Design review of the part built by this model. Coordinates are the model's own, in mm. Face numbers are marked on the shaded views. A direction names the side the tool comes from. Give positions to 0.01 mm unless a question says otherwise; leave off trailing zeros. Loops run counter-clockwise (first coordinate to the right, second up) from the corner with the lowest first, then second, coordinate; pieces in that order, holes last. Notation, with made-up numbers: M 64.25,73.5 L 87.25,73.5 A34 ccw 87.25,108.5 Z; hole C 56.25,12.25 d4. An arc over 180 degrees is marked long. Answer as CSV lines item,"result".
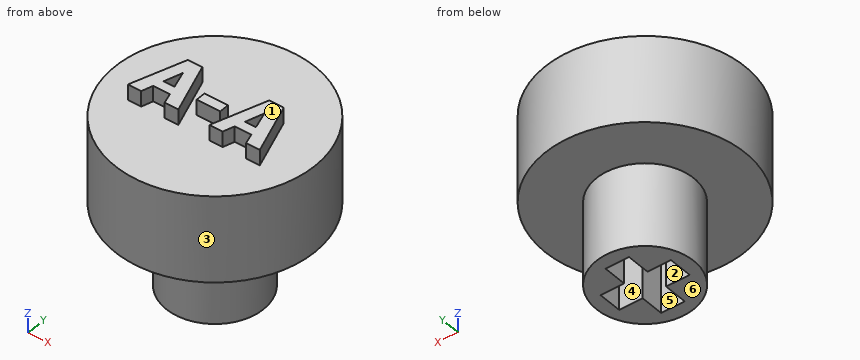
Autodesk Inventor part; units mm, degrees
ref_plane "YZ Plane" through (0, 0, 0) normal (1, 0, 0) x (0, 1, 0)
ref_plane "XZ Plane" through (0, 0, 0) normal (0, 1, 0) x (-1, 0, 0)
ref_plane "XY Plane" through (0, 0, 0) normal (0, 0, 1) x (1, 0, 0)
sketch "Sketch1" plane through (0, 0, 0) normal (0, 0, 1) x (1, 0, 0)
  circle A0 centre (0, 0) radius 6.22 construction
  circle A1 centre (0, 0) radius 2.8
  line L0 (-0.675, 0.675) -> (-0.675, 2.025)
  line L1 (-0.675, 2.025) -> (0.675, 2.025)
  line L2 (0.675, 2.025) -> (0.675, 0.675)
  line L3 (0.675, 0.675) -> (2.025, 0.675)
  line L4 (2.025, 0.675) -> (2.025, -0.675)
  line L5 (2.025, -0.675) -> (0.675, -0.675)
  line L6 (0.675, -0.675) -> (0.675, -2.025)
  line L7 (0.675, -2.025) -> (-0.675, -2.025)
  line L8 (-0.675, -2.025) -> (-0.675, -0.675)
  line L9 (-0.675, -0.675) -> (-2.025, -0.675)
  line L10 (-2.025, -0.675) -> (-2.025, 0.675)
  line L11 (-2.025, 0.675) -> (-0.675, 0.675)
  circle A2 centre (0, 0) radius 5.75
  point P0 (-6.07, -6.1)
  dimension "d0" = 12.44
  dimension "d1" = 0.47
extrude "Extrusion1" add sketch "Sketch1" along normal blind 5 contours A1 | L0 L1 L2 L3 L4 L5 L6 L7 L8 L9 L10 L11 | A2
extrude "Extrusion2" add sketch "Sketch1" against normal blind 4.8 contours A1
sketch "Sketch2" plane through (0, 0, 5) normal (0, 0, 1) x (1, 0, 0)
  point P0 (0, 0)
sketch "Sketch3" plane through (0, 0, 5) normal (0, 0, 1) x (1, 0, 0)
  line L0 (-3.7906, 1.533) -> (3.7906, 1.533) construction
  line L1 (3.7906, 1.533) -> (3.7906, -1.533) construction
  line L2 (3.7906, -1.533) -> (-3.7906, -1.533) construction
  line L3 (-3.7906, -1.533) -> (-3.7906, 1.533) construction
  line L4 (-3.803, -1.517) -> (-2.7723, 1.533)
  line L5 (-2.7723, 1.533) -> (-1.9369, 1.533)
  line L6 (-1.9369, 1.533) -> (-0.9062, -1.517)
  line L7 (-0.9062, -1.517) -> (-1.6947, -1.517)
  line L8 (-1.6947, -1.517) -> (-1.885, -0.8941)
  line L9 (-1.885, -0.8941) -> (-2.844, -0.8941)
  line L10 (-2.844, -0.8941) -> (-3.0368, -1.517)
  line L11 (-3.0368, -1.517) -> (-3.803, -1.517)
  line L12 (-2.0531, -0.3405) -> (-2.3645, 0.6679)
  line L13 (-2.3645, 0.6679) -> (-2.6784, -0.3405)
  line L14 (-2.6784, -0.3405) -> (-2.0531, -0.3405)
  line L15 (0.6633, -0.4542) -> (-0.6937, -0.4542)
  line L16 (-0.6937, -0.4542) -> (-0.6937, 0.1143)
  line L17 (-0.6937, 0.1143) -> (0.6633, 0.1143)
  line L18 (0.6633, 0.1143) -> (0.6633, -0.4542)
  line L19 (0.8783, -1.517) -> (1.909, 1.533)
  line L20 (1.909, 1.533) -> (2.7444, 1.533)
  line L21 (2.7444, 1.533) -> (3.7751, -1.517)
  line L22 (3.7751, -1.517) -> (2.9866, -1.517)
  line L23 (2.9866, -1.517) -> (2.7963, -0.8941)
  line L24 (2.7963, -0.8941) -> (1.8373, -0.8941)
  line L25 (1.8373, -0.8941) -> (1.6445, -1.517)
  line L26 (1.6445, -1.517) -> (0.8783, -1.517)
  line L27 (2.6282, -0.3405) -> (2.3168, 0.6679)
  line L28 (2.3168, 0.6679) -> (2.0029, -0.3405)
  line L29 (2.0029, -0.3405) -> (2.6282, -0.3405)
  point P0 (0, -1.533)
  point P1 (3.7906, 0)
  point P2 (0, 0)
  point P3 (0, 0)
extrude "Extrusion6" add sketch "Sketch3" along normal blind 0.9
properties part number "IPC A-A key"
1. We need section B-B, the plane x = 0. Write out the cut boundary in (y, z) (3 decimals).
Answer block:
outline,"M -5.75,0 L -2.8,0 L -2.8,-4.8 L -2.025,-4.8 L -2.025,0 L 2.025,0 L 2.025,-4.8 L 2.8,-4.8 L 2.8,0 L 5.75,0 L 5.75,5 L 0.114,5 L 0.114,5.9 L -0.454,5.9 L -0.454,5 L -5.75,5 Z"
2. The part is to be moulded in two halves that separate along X. For the marked faces 3, 4, 5 and 6, say which applies: pulls with the +X half, pulls with the -X half, needs draft (parallel to the pull), parting line crosses it, or undercut.
Answer block:
face 3,"parting line crosses it"
face 4,"undercut"
face 5,"undercut"
face 6,"needs draft"
3. We need section D-D, the plane y = 3.75. Write out the cut boundary in (x, z).
Answer block:
outline,"M -4.36,0 L 4.36,0 L 4.36,5 L -4.36,5 Z"
4. To check wall thickness, follow L1, parallel to Z at x = 4.75, y = -1; L2, parallel to Z at x = 2, y = -1.5; L3, parallel to X at y = -0.5, z = -3 (3 decimals). State the ranges of each line that lie inside material, in increasing order. Write a range as [from, to].
Answer block:
L1,"[0, 5]"
L2,"[-4.8, 5]"
L3,"[-2.755, -2.025], [2.025, 2.755]"
5. For the marked faces 1 and 2, list the 3-axis set-ups (+Z, -Z, +X, -X, +Y, -Y) from which the entire face can be reached by the end or side of a thin tool; tool diameter is ignored.
Answer block:
face 1,"+Z, +X, -X, +Y, -Y"
face 2,"-Z"
6. We need section C-C, the plane z = 2.75. Write out the cut boundary in (x, y), plus the area to 3 significant figures.
Answer block:
outline,"C 0,0 d11.5"
area,"104 mm²"
7. For P1, Ø0.9, axis at x = 3.5, z = 5.5, coming from the -Y side; P2, Ø0.7, axis at x = 0, z = 5.5, coming from the -Y side; P3, Ø1.1, axis at x = 1.5, z = -3.5, coming from the -Y side, all flat-tipped, find the tip position at first contact; note any pin that passes through.
Answer block:
P1,"y = -1.52"
P2,"y = -0.45"
P3,"y = -2.63"
8. We need section A-A, the plane z = -3.5. Write out the cut boundary in (x, y) (3 decimals), plus the area to 3 significant figures.
Answer block:
outline,"C 0,0 d5.6; hole M -2.025,-0.675 L -0.675,-0.675 L -0.675,-2.025 L 0.675,-2.025 L 0.675,-0.675 L 2.025,-0.675 L 2.025,0.675 L 0.675,0.675 L 0.675,2.025 L -0.675,2.025 L -0.675,0.675 L -2.025,0.675 Z"
area,"15.5 mm²"
